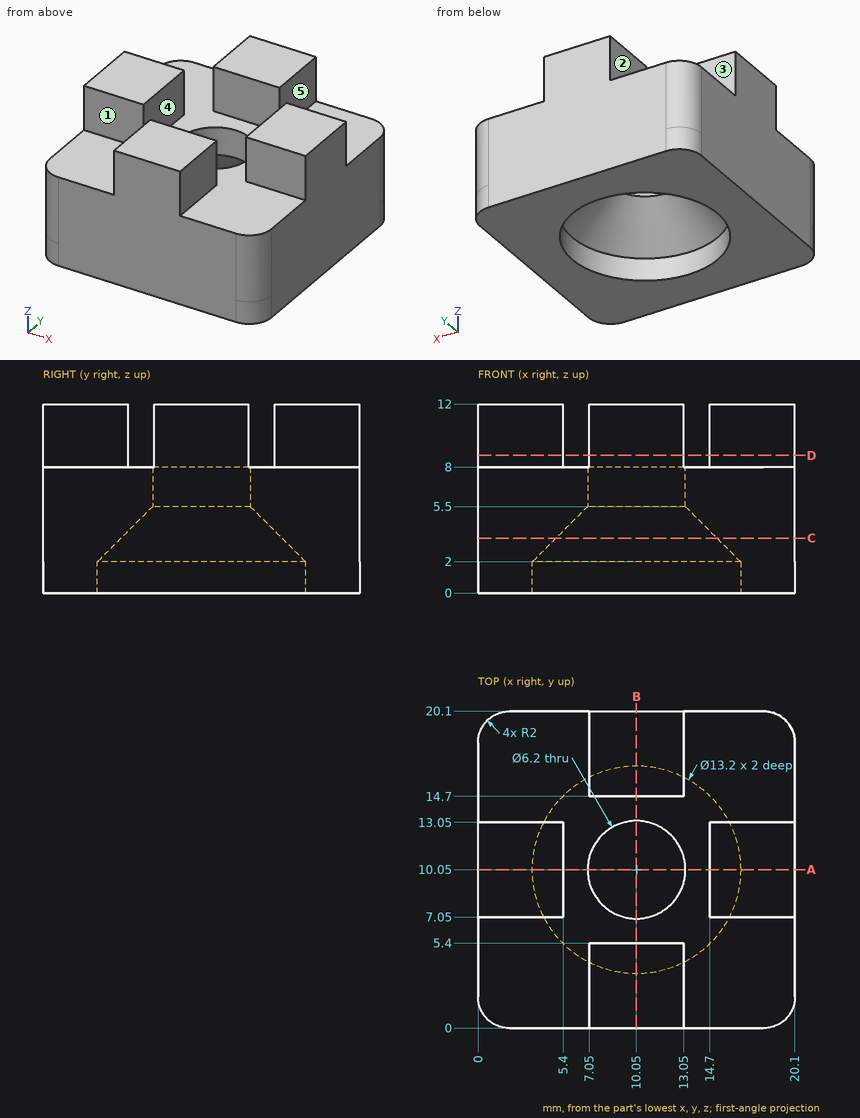
Verification items for this drawing (mm, ordinates from the low corner). A direction names the side the tool comes from. Coordinates: 2 decimals unless noted, no trailing zeros. Order: outer loops, then holes, each group sorted by start corner. A loop starts at its lowest first (then second) coordinate and runs counter-clockwise, first axis right, second up.
Q1. Sectioned sample at C-C on z = 3.5. Record the cut outline in (x, y), and give its area (3 significant figures).
Reply:
outline: (0, 2) arc R2 ccw to (2, 0) - (18.1, 0) arc R2 ccw to (20.1, 2) - (20.1, 18.1) arc R2 ccw to (18.1, 20.1) - (2, 20.1) arc R2 ccw to (0, 18.1) - close; hole circle Ø10.2 at (10.05, 10.05)
area: 319 mm2
Q2. Thickness scan on probe 1 along Y at (x, z) = (10.05, 0.4); probe 2 along Z at (x, y) = (14.5, 15.5); probe 3 along Y at (x, z) = (14, 1). Record the ranges inside material, lowest first.
Reply:
probe 1: y = 0 to 3.45, 16.65 to 20.1
probe 2: z = 0 to 8
probe 3: y = 0 to 4.76, 15.34 to 20.1
Q3. Tool access check on the marked faces 1, 2, 3, 4 and 5. Record the directions out of +Z, -Z, +X, -X, +Y, -Y that give a thin tool (end or side, any length) a straight path to the whole face; none if there is none.
Reply:
face 1: +Z, +X, -X, -Y
face 2: +Z, -X, +Y, -Y
face 3: +Z, +X, -X, +Y
face 4: +Z, +Y, -Y
face 5: +Z, +X, +Y, -Y
Q4. Sectioned sample at A-A on y = 10.05. Record the cut outline in (x, z), and give its area (3 significant figures).
Reply:
outline: (0, 0) - (3.45, 0) - (3.45, 2) - (6.95, 5.5) - (6.95, 8) - (5.4, 8) - (5.4, 12) - (0, 12) - close; (13.15, 5.5) - (16.65, 2) - (16.65, 0) - (20.1, 0) - (20.1, 12) - (14.7, 12) - (14.7, 8) - (13.15, 8) - close
area: 128 mm2
Q5. Sectioned sample at D-D on z = 8.75. Record the cut outline in (x, y).
Reply:
outline: (0, 7.05) - (5.4, 7.05) - (5.4, 13.05) - (0, 13.05) - close; (7.05, 0) - (13.05, 0) - (13.05, 5.4) - (7.05, 5.4) - close; (7.05, 14.7) - (13.05, 14.7) - (13.05, 20.1) - (7.05, 20.1) - close; (14.7, 7.05) - (20.1, 7.05) - (20.1, 13.05) - (14.7, 13.05) - close
Q6. Depth check by flat-ended pin: pin 1 Ø3 at (y, z) = (17, 11) entering from -X; pin 2 Ø3.5 at (x, y) = (10.05, 10.05) entering from +Z; pin 3 Ø2 at (x, z) = (18, 9.5) entering from -Y; pin 4 Ø1.2 at (x, z) = (3.5, 11) entering from +Y. Enter the tip coordinate at first touch or a pass-through.
Reply:
pin 1: stops at x = 7.05
pin 2: passes through
pin 3: stops at y = 7.05
pin 4: stops at y = 13.05
